Source: three-view drawing plus pictorial views. Frame: mm from the lowest corner of the part. A direction names the side the tool comes from. Give positions to 0.01 mm unless a question says otherwise; leave off trailing zeros. Order: outer loops, then holes, each group sorted by start corner. A loop starts at its lowest first (then second) coordinate and runs counter-clockwise, first axis right, second up. Notation, with made-up numbers: M 87.25,65 L 95.25,65 A29 cw 95.25,86 Z; hole C 12,45 d11. An arc over 180 degrees is marked long. Use CSV: the item, a comma, the result in double quotes. Start each with the question number.
Item 1: Section query D-D on x = 18.75. Return loops of the section in (y, z).
Item 2: Access query for the marked faces 4, 5 and 6. Directions: +Z, -Z, +X, -X, +Y, -Y. A direction counts if a zero-diameter tool reaches every point of the face in a straight line with its end or side. Return the directions, or none.
Item 3: Pull-direction query (Z, two-part tool) for the marked faces 1, 2 and 3; classes: +Z half, -Z half, draft (parallel to the pull), parting line (faces both ways), or undercut.
Item 4: Ray query, probe 1 along Z at (x, y) = (19.15, 4); probe 2 along Y at (x, z) = (18.75, 13.5); probe 3 along X at (y, z) = (13, 9.75). Return the intervals inside material, ascending. Write a range as from..to.
Item 5: First-contact query: pin 1 (4 mm diameter, centred on x = 7, y = 5, fed in from -Z); pin 2 (5 mm diameter, centred on y = 16, z = 13, fed in from -X). Flat tips, straight axial feed; report the tip coordinate or a pass-through.
Item 6: Section query A-A on z = 9.5. Return loops of the section in (x, y), and give its area (3 significant figures).
Item 7: Section query C-C on z = 14. Return loops of the section in (x, y), and give its area (3 significant figures).
Item 8: Section query B-B on y = 29. Return loops of the section in (x, z).
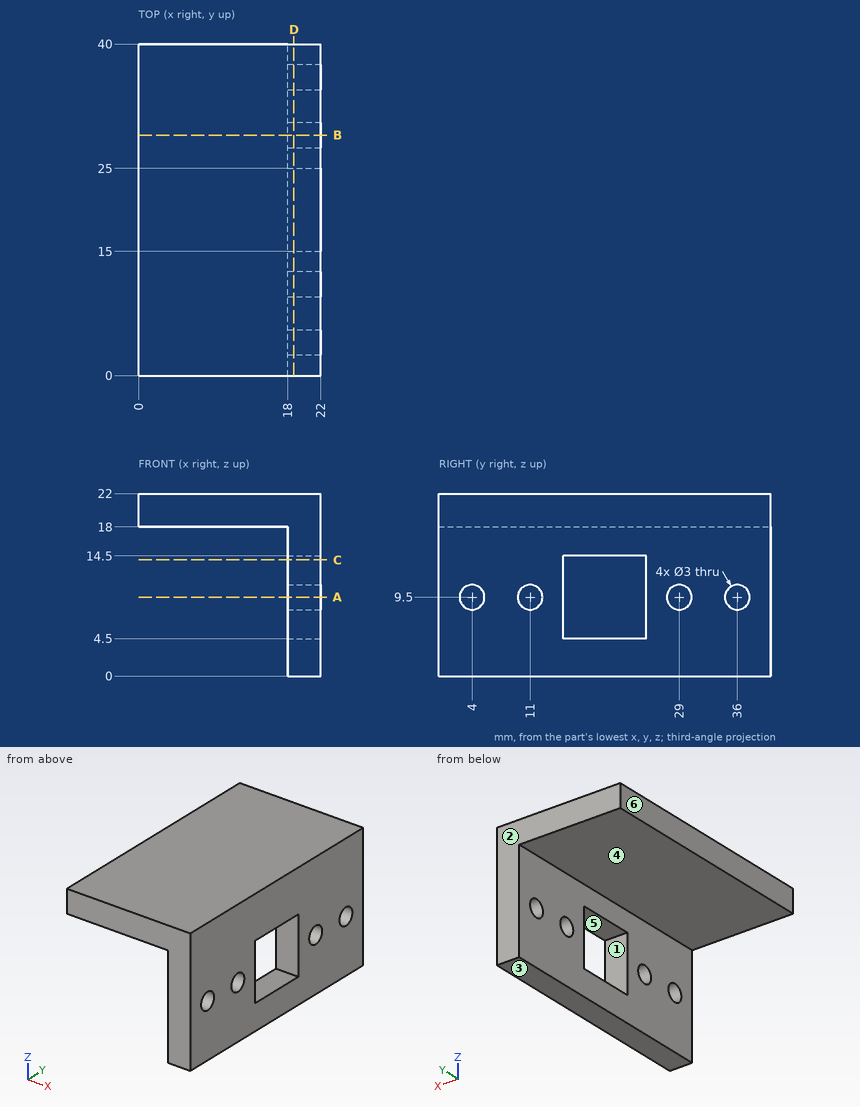
Verdict:
1,outline,"M 0,0 L 40,0 L 40,22 L 0,22 Z; hole C 4,9.5 d3; hole C 11,9.5 d3; hole M 15,4.5 L 25,4.5 L 25,14.5 L 15,14.5 Z; hole C 29,9.5 d3; hole C 36,9.5 d3"
2,face 4,"-Z, -X, +Y, -Y"
2,face 5,"+X, -X"
2,face 6,"+Z, -Z, -X, +Y, -Y"
3,face 1,"undercut"
3,face 2,"draft"
3,face 3,"-Z half"
4,probe 1,"0..8, 11..22"
4,probe 2,"0..15, 25..40"
4,probe 3,"18..22"
5,pin 1,"z = 18"
5,pin 2,"x = 18"
6,outline,"M 18,0 L 22,0 L 22,2.5 L 18,2.5 Z; M 18,5.5 L 22,5.5 L 22,9.5 L 18,9.5 Z; M 18,12.5 L 22,12.5 L 22,15 L 18,15 Z; M 18,25 L 22,25 L 22,27.5 L 18,27.5 Z; M 18,30.5 L 22,30.5 L 22,34.5 L 18,34.5 Z; M 18,37.5 L 22,37.5 L 22,40 L 18,40 Z"
6,area,"72.0 mm2"
7,outline,"M 18,0 L 22,0 L 22,15 L 18,15 Z; M 18,25 L 22,25 L 22,40 L 18,40 Z"
7,area,"120 mm2"
8,outline,"M 0,18 L 18,18 L 18,11 L 22,11 L 22,22 L 0,22 Z; M 18,0 L 22,0 L 22,8 L 18,8 Z"
